Can you work these out from the model? Positions are in its coordinate system, mm. A direction names the side the tool comes from. Give positions to 0.01 mm unless a question says otherwise; leave off trailing zeros. Order: outer loops, then holes, each group sorted by start corner. A loop starts at its lowest first (then second) coordinate and runs counter-clockwise, first axis right, second up.
Item 1: I want a section at C-C, the plane z = 3.35. Write out the boundary of the cut face in (x, y), then the cut area to 3 significant figures.
Item 2: Which directions (+Z, -Z, +X, -X, +Y, -Y) give clear straight access to the entire face, cutting with the end or side of a thin tool? Please do faces 5 (the flat face through (20.55, 26, 3)), 6 (the flat face through (32.05, 26, 3)).
Item 3: I want a section at B-B, the plane x = 25.5. Write out the boundary of the cut face in (y, z), then the cut area to 3 significant figures.
Item 4: If I drill on line 1 along X through (y, z) = (22, 1.25); line 2 along Y through (x, z) = (20.75, 2.7), over which ranges is the centre line in solid material (lowest first)?
Item 5: If we mould it in two halves opening along Y, with no side actions, what happens to faces 1 (the flat face through (25, 21.8, 3)), 2 (the flat face through (25, 20, 3)), 3 (the flat face through (30.25, 26, 3)), 4 (the flat face through (18.75, 26, 3))? For each: +Y half, -Y half, draft (parallel to the pull), parting line (faces both ways), or undercut.
Item 6: I want a section at A-A, the plane y = 22.5. Write out the boundary of the cut face in (x, z).
```python
from build123d import *

# Parameters (mm, degrees)
BOX004_W     = 9.7
BOX004_H     = 9.3
BOX004_DEPTH = 5.1
BOX005_W     = 13.3
BOX005_H     = 12.9
BOX005_DEPTH = 5.1


with BuildPart() as cube004:
    # Box004 → Box004 (new body)
    with BuildSketch(Plane(origin=(1.8, 1.8, 0), x_dir=(1, 0, 0), z_dir=(0, 0, 1))):
        with Locations((4.85, 4.65)):
            Rectangle(BOX004_W, BOX004_H)
    extrude(amount=BOX004_DEPTH)


with BuildPart() as cut001:
    # Box005 → Box005 (new body)
    with BuildSketch(Plane.XY):
        with Locations((6.65, 6.45)):
            Rectangle(BOX005_W, BOX005_H)
    extrude(amount=BOX005_DEPTH)

    # Cut001: cut Cube004
    add(cube004.part, mode=Mode.SUBTRACT)


with BuildPart() as cut001_1:
    # Cut001 placement: moved
    add(cut001.part.moved(Location((18.75, 20, 0))))


solid = cut001_1.part
```
Results list:
1. outline: (18.75, 20) - (32.05, 20) - (32.05, 32.9) - (18.75, 32.9) - close; hole (20.55, 21.8) - (30.25, 21.8) - (30.25, 31.1) - (20.55, 31.1) - close
1. area: 81.4 mm2
2. face 5: +Z, -Z
2. face 6: +Z, -Z, +X, +Y, -Y
3. outline: (20, 0) - (21.8, 0) - (21.8, 5.1) - (20, 5.1) - close; (31.1, 0) - (32.9, 0) - (32.9, 5.1) - (31.1, 5.1) - close
3. area: 18.4 mm2
4. line 1: x = 18.75 to 20.55, 30.25 to 32.05
4. line 2: y = 20 to 21.8, 31.1 to 32.9
5. face 1: undercut
5. face 2: -Y half
5. face 3: undercut
5. face 4: draft
6. outline: (18.75, 0) - (20.55, 0) - (20.55, 5.1) - (18.75, 5.1) - close; (30.25, 0) - (32.05, 0) - (32.05, 5.1) - (30.25, 5.1) - close
